```python
from build123d import *

# Parameters (mm, degrees)
SKETCH1_W           = 17.5
SKETCH1_H           = 17.5
BOSS_EXTRUDE1_DEPTH = 20
SKETCH2_W           = 11.5
SKETCH2_H           = 11.5
CUT_EXTRUDE1_DEPTH  = 17
SKETCH4_W           = 4
SKETCH4_H           = 17.5
BOSS_EXTRUDE2_DEPTH = 2
LPATTERN1_COUNT     = 8
LPATTERN1_PITCH     = 19.5
SKETCH5_W           = 16
SKETCH5_H           = 17.5
BOSS_EXTRUDE3_DEPTH = 2
SKETCH6_W           = 20
SKETCH6_H           = 17.5
BOSS_EXTRUDE4_DEPTH = 2
SKETCH7_W           = 125
SKETCH7_H           = 2.5
CUT_EXTRUDE2_DEPTH  = 2
SKETCH8_W           = 156
SKETCH8_H           = 15.5
SKETCH8_W_2         = 152.631082986
SKETCH8_H_2         = 13.5
BOSS_EXTRUDE5_DEPTH = 2
SKETCH9_W           = 156
SKETCH9_H           = 15.5
BOSS_EXTRUDE6_DEPTH = 2
SKETCH10_W          = 158
SKETCH10_H          = 17.5
BOSS_EXTRUDE7_DEPTH = 5


with BuildPart() as part:
    # Sketch1 → Boss-Extrude1 (new body)
    with BuildSketch(Plane.XY):
        with Locations((8.75, 8.75)):
            Rectangle(SKETCH1_W, SKETCH1_H)
    extrude(amount=BOSS_EXTRUDE1_DEPTH)

    # Sketch2 → Cut-Extrude1 (cut)
    with BuildSketch(Plane.XY.offset(20)):
        with Locations((8.75, 8.75)):
            Rectangle(SKETCH2_W, SKETCH2_H)
    extrude(amount=-CUT_EXTRUDE1_DEPTH, mode=Mode.SUBTRACT)

    # Sketch4 → Boss-Extrude2 (add)
    with BuildSketch(Plane.ZY):
        with Locations((18, 8.75)):
            Rectangle(SKETCH4_W, SKETCH4_H)
    extrude(amount=BOSS_EXTRUDE2_DEPTH)


with BuildPart() as lpattern1_1:
    # LPattern1: pattern copy
    add(part.part.moved(Location(Vector(-1, 0, 0) * (1 * LPATTERN1_PITCH))))


with BuildPart() as lpattern1_2:
    # LPattern1: pattern copy
    add(part.part.moved(Location(Vector(-1, 0, 0) * (2 * LPATTERN1_PITCH))))


with BuildPart() as lpattern1_3:
    # LPattern1: pattern copy
    add(part.part.moved(Location(Vector(-1, 0, 0) * (3 * LPATTERN1_PITCH))))


with BuildPart() as lpattern1_4:
    # LPattern1: pattern copy
    add(part.part.moved(Location(Vector(-1, 0, 0) * (4 * LPATTERN1_PITCH))))


with BuildPart() as lpattern1_5:
    # LPattern1: pattern copy
    add(part.part.moved(Location(Vector(-1, 0, 0) * (5 * LPATTERN1_PITCH))))


with BuildPart() as lpattern1_6:
    # LPattern1: pattern copy
    add(part.part.moved(Location(Vector(-1, 0, 0) * (6 * LPATTERN1_PITCH))))


with BuildPart() as lpattern1_7:
    # LPattern1: pattern copy
    add(part.part.moved(Location(Vector(-1, 0, 0) * (7 * LPATTERN1_PITCH))))


with BuildPart() as lpattern1_4_1:
    add(lpattern1_4.part)

    # Combine1: union LPattern1_5, LPattern1_6, LPattern1_7, LPattern1_1, LPattern1_2, part, LPattern1_3
    add(lpattern1_5.part)
    add(lpattern1_6.part)
    add(lpattern1_7.part)
    add(lpattern1_1.part)
    add(lpattern1_2.part)
    add(part.part)
    add(lpattern1_3.part)

    # Sketch5 → Boss-Extrude3 (add)
    with BuildSketch(Plane.ZY.offset(136.5)):
        with Locations((8, 8.75)):
            Rectangle(SKETCH5_W, SKETCH5_H)
    extrude(amount=BOSS_EXTRUDE3_DEPTH)

    # Sketch6 → Boss-Extrude4 (add)
    with BuildSketch(Plane(origin=(17.5, 0, 0), x_dir=(0, 0, -1), z_dir=(1, 0, 0))):
        with Locations((-10, 8.75)):
            Rectangle(SKETCH6_W, SKETCH6_H)
    extrude(amount=BOSS_EXTRUDE4_DEPTH)

    # Sketch7 → Cut-Extrude2 (cut)
    with BuildSketch(Plane.XY.offset(20)):
        with Locations((-59.5, 8.75)):
            Rectangle(SKETCH7_W, SKETCH7_H)
    extrude(amount=-CUT_EXTRUDE2_DEPTH, mode=Mode.SUBTRACT)

    # Sketch8 → Boss-Extrude5 (add)
    with BuildSketch(Plane.XY.offset(20)):
        with Locations((-59.5, 8.75)):
            Rectangle(SKETCH8_W, SKETCH8_H)
        with Locations((-59.5, 8.75)):
            Rectangle(SKETCH8_W_2, SKETCH8_H_2, mode=Mode.SUBTRACT)
    extrude(amount=BOSS_EXTRUDE5_DEPTH)

    # Sketch9 → Boss-Extrude6 (add)
    with BuildSketch(Plane.XY.offset(20)):
        with Locations((-59.5, 8.75)):
            Rectangle(SKETCH9_W, SKETCH9_H)
    extrude(amount=BOSS_EXTRUDE6_DEPTH)

    # Sketch10 → Boss-Extrude7 (add)
    with BuildSketch(Plane.XY.offset(20)):
        with Locations((-59.5, 8.75)):
            Rectangle(SKETCH10_W, SKETCH10_H)
    extrude(amount=BOSS_EXTRUDE7_DEPTH)


solid = lpattern1_4_1.part
```
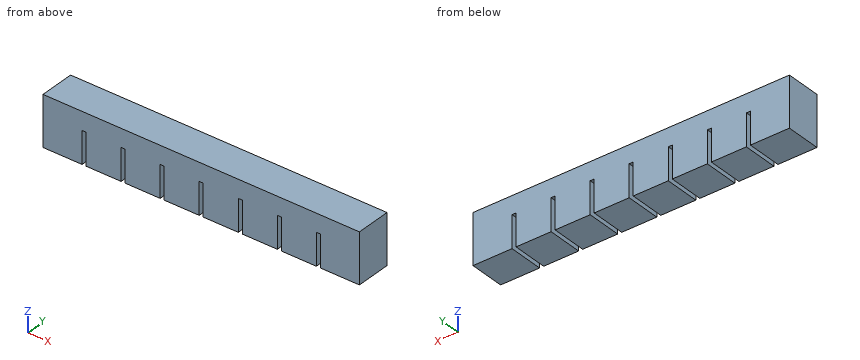
For this review, take the finished solid that the model builds, in its own axes (mm). Round coordinates to 2 decimals unless told otherwise and drop trailing zeros. Write each loop counter-clockwise with the first axis right and the second up, starting at its lowest first coordinate (ties: lowest second). Pieces come first, ordered by that corner, then holes.
1) For line 1 along Y through (x, z) = (-64, 7); line 2 along Z through (x, y) = (-130, 8.75), list the stretches that pass through material, from the lowest coordinate up.
Answer below:
line 1: y = 0 to 3, 14.5 to 17.5
line 2: z = 0 to 3, 20 to 25
2) Insertion check: pin 1 Ø1 at (x, y) = (-79, 13) entering from -Z. The pin has a flat end and moves straight along its axis. Give the tip position at first contact, or say it passes through.
Answer below:
pin 1: stops at z = 16
3) Take a section at A-A on z = 13. State how many separate pieces and enclosed holes the cut face has, then the cut area to 3 significant figures.
Answer below:
separate pieces: 8
enclosed holes: 8
area: 1,460 mm2
4) Take a section at B-B on x = -109. Give the boundary of the cut face in (y, z).
Answer below:
outline: (0, 0) - (17.5, 0) - (17.5, 25) - (0, 25) - close; hole (3, 3) - (14.5, 3) - (14.5, 20) - (3, 20) - close
